from build123d import *

# Parameters (mm, degrees)
F2_R     = 4.7625
F3_DEPTH = 9.525


with BuildPart() as f1:
    # F0 (on Front) → F1 (revolve)
    with BuildSketch(Plane.XZ):
        with BuildLine():
            Line((0, 50.8), (0, 0))
            Line((0, 0), (10.261248, 0))
            Line((10.261248, 0), (21.929258, 7.154912))
            ThreePointArc((21.929258, 7.154912), (24.1506, 9.46627), (24.959791, 12.568196))
            Line((24.959791, 12.568196), (24.959791, 17.333189))
            Line((24.959791, 17.333189), (10.261248, 17.333189))
            Line((10.261248, 17.333189), (10.261248, 50.8))
            Line((10.261248, 50.8), (0, 50.8))
        make_face()
    revolve(axis=Axis((0, 0, 25.4), (0, 0, 1)))

    # F2 (on face) → F3 (cut)
    with BuildSketch(Plane.XY.offset(50.8)):
        Circle(F2_R)
    extrude(amount=-F3_DEPTH, mode=Mode.SUBTRACT)


solid = f1.part
CAD build for the part. Positions are in the model's coordinates, mm. A direction names the side the tool comes from. Give positions to 0.01 mm unless a question says otherwise; leave off trailing zeros. Order: outer loops, then holes, each group sorted by start corner. A loop starts at its lowest first (then second) coordinate and runs counter-clockwise, first axis right, second up. Notation, with made-up numbers: (49, 47.25) - (84, 47.25) arc R27 cw to (84, 69.25) - close; hole circle Ø6 at (66, 47.25). An arc over 180 degrees is marked (long way). Answer in a Markdown table with one row per item.
1. Saw through at D-D, the plane z = 20. Give the cut face in (x, y).
Data:
| item | result |
|---|---|
| outline | circle Ø20.52 at (0, 0) |
2. Tool access for faces 5 (the conical face through (-1.43, 10.9, 0.45)), 6 (the cylindrical face through (-8.143, -6.244, 34.301)): list every direction of +Z, -Z, +X, -X, +Y, -Y with a clear straight run to the whole face (end or side of a thin tool).
Data:
| item | result |
|---|---|
| face 5 | -Z |
| face 6 | +Z |
3. Flat gauge pins, fed straight in: pin 1 (8 mm diameter, centred on y = -14, z = 13.5, fed in from -X); pin 2 (8 mm diameter, centred on x = -12.5, z = 15, fed in from +Y); pin 3 (1 mm diameter, centred on x = -10.5, y = -11, fed in from -Z). Where does each tip first touch, or does it go through?
Data:
| item | result |
|---|---|
| pin 1 | stops at x = -22.87 |
| pin 2 | stops at y = 23.47 |
| pin 3 | stops at z = 2.73 |
4. Probe probe 1 along Y at (x, z) = (0, 46.5); probe 2 along X at (y, z) = (-21, 12); probe 3 along Z at (x, y) = (-2, -2.5) (3 decimals). List the from-to ranges inside material, lowest first. Write a range as [from, to].
Data:
| item | result |
|---|---|
| probe 1 | y = [-10.26, -4.76], [4.76, 10.26] |
| probe 2 | x = [-13.44, 13.44] |
| probe 3 | z = [0, 41.275] |
5. Pull direction X, two halves, no side cores. Call faces 1 (the flat face through (0, 0, 41.275)), 2 (the flat face through (4.4, 2.4, 50.8)), 3 (the cylindrical face through (-3.78, -2.9, 46.1)), 4 (the cylindrical face through (-3.249, 24.747, 14.984)): pulls with the +X half, pulls with the -X half, needs draft (parallel to the pull), parting line crosses it, or undercut.
Data:
| item | result |
|---|---|
| face 1 | undercut |
| face 2 | needs draft |
| face 3 | undercut |
| face 4 | parting line crosses it |
6. Saw through at C-C, the plane z = 42. Give the cut face in (x, y) (1 decimal), plus the area to 3 significant figures.
Data:
| item | result |
|---|---|
| outline | circle Ø20.5 at (0, 0); hole circle Ø9.5 at (0, 0) |
| area | 260 mm² |
